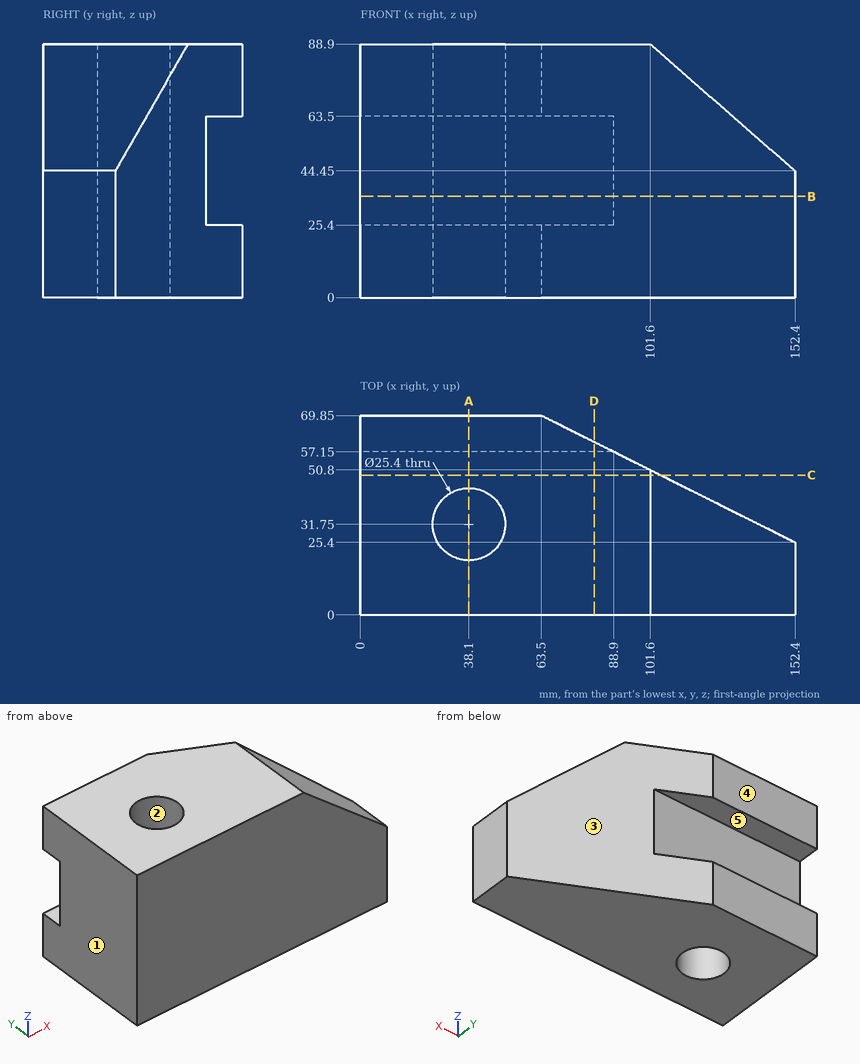
Geometry: see drawing. Coordinates: mm, zero at the bounding-box minimum. A direction names the side the tool comes from. Coordinates: 2 decimals unless noted, no trailing zeros. Loops run counter-clockwise (first coordinate to the right, second up) from the corner with the lowest first, then second, coordinate; pieces in that order, holes last.
Q1. Draft query along Y for the marked faces 1, 2 and 3. Return one class per face: +Y half, -Y half, draft (parallel to the pull), parting line (faces both ways), or undercut.
Q2. Cut plane C-C (y = 49). Output: boundary loops of the cut face in (x, z), then the cut area to 3 significant figures.
Q3. Contact query for flat-ended pins moving along their axis: pin 1 (5 mm diameter, centred on y = 53, z = 37.5, fed in from -X); pin 2 (12 mm diameter, centred on x = 109.5, z = 48, fed in from +Y); pin 3 (10 mm diameter, centred on x = 121.5, z = 26, fed in from +Y). Output: stop coordinate, or through.
Q4. Set-up query: the marked faces 4 and 5. Return all of +Z, -Z, +X, -X, +Y, -Y with unobstructed straight access to the full face (end or side cutting, diameter ignored); none if empty.
Q5. Cut plane D-D (x = 82). Output: boundary loops of the cut face in (y, z), then the cut area to 3 significant figures.
Q6. Material intervals for line 1 (Y direction, x = 38, z = 27); line 2 (Y direction, x = 38.1, z = 21.5); line 3 (Z direction, x = 33, y = 61.5), sorted ascending.
Q7. Cut plane B-B (z = 35.5). Output: boundary loops of the cut face in (x, y).
Q8. Cut plane A-A (x = 38.1). Output: boundary loops of the cut face in (y, z), then the cut area to 3 significant figures.
Working result:
1. face 1: draft
1. face 2: undercut
1. face 3: +Y half
2. outline: (0, 0) - (105.2, 0) - (105.2, 85.75) - (101.6, 88.9) - (0, 88.9) - close
2. area: 9,350 mm2
3. pin 1: stops at x = 0
3. pin 2: stops at y = 49.85
3. pin 3: stops at y = 43.35
4. face 4: +Z, -Z, +X, -X, +Y
4. face 5: +X, -X, +Y
5. outline: (0, 0) - (60.6, 0) - (60.6, 25.4) - (57.15, 25.4) - (57.15, 63.5) - (60.6, 63.5) - (60.6, 88.9) - (0, 88.9) - close
5. area: 5,260 mm2
6. line 1: y = 0 to 19.05, 44.45 to 57.15
6. line 2: y = 0 to 19.05, 44.45 to 69.85
6. line 3: z = 0 to 25.4, 63.5 to 88.9
7. outline: (0, 0) - (152.4, 0) - (152.4, 25.4) - (88.9, 57.15) - (0, 57.15) - close; hole circle Ø25.4 at (38.1, 31.75)
8. outline: (0, 0) - (19.05, 0) - (19.05, 88.9) - (0, 88.9) - close; (44.45, 0) - (69.85, 0) - (69.85, 25.4) - (57.15, 25.4) - (57.15, 63.5) - (69.85, 63.5) - (69.85, 88.9) - (44.45, 88.9) - close
8. area: 3,470 mm2
